Can you work these out from the model? Positions are in its coordinate system, mm. A direction names the side the tool comes from. Coordinates: 2 decimals unless noted, no trailing zeros. Write each loop counter-clockwise with the first axis right and the second up, starting at its lowest first coordinate (ties: lowest second). Pieces come first, ordered by that corner, then holes. Notation, with made-up numbers: (-22.5, 2.5) -> (0.5, 2.5) arc R16 cw to (0.5, 9.5) -> close; hole circle Ø7 at (78, 83.25). An arc over 180 degrees is marked (long way). Answer as CSV lines item,"result". Start each with the question number.
Autodesk Inventor part; units mm, degrees
ref_plane "YZ Plane" through (0, 0, 0) normal (1, 0, 0) x (0, 1, 0)
ref_plane "XZ Plane" through (0, 0, 0) normal (0, 1, 0) x (-1, 0, 0)
ref_plane "XY Plane" through (0, 0, 0) normal (0, 0, 1) x (1, 0, 0)
sketch "Sketch1" plane through (0, 0, 0) normal (0, 1, 0) x (-1, 0, 0)
  circle A0 centre (0, 0) radius 25.4
  dimension "d0" = 50.8
extrude "Extrusion1" add sketch "Sketch1" against normal blind 25.4
fillet "Fillet1" radius 6.35 1 edges at (25.4, -25.4, 0)
hole "Hole1" at (0, -25.4, 0) direction (0, 1, 0) diameter 6.7564 end through all counterbore diameter 11.1252 counterbore depth 6.35
properties part number "foot"
Q1. Which directions (+Z, -Z, +X, -X, +Y, -Y) give clear straight access to the entire face, cutting with the end or side of a thin tool? Please do faces 1 (the face through (-1.671, -22.181, -5.306)), 2 (the face through (-5, 0, 0)).
Q2. If we mould it in two halves opening along X, with no side actions, what happens to faces 3 (the face through (-4, -25.4, 5)), 4 (the face through (5.506, -9.392, -24.796)), 5 (the face through (0, -19.05, -4))? For each: released by +X, released by -X, zero draft, split by the parting line, or undercut.
Q3. I need wall thicknesses on L1, parallel to Z at x = 0, y = -6.75; L2, parallel to Z at x = 2, y = -19.5; L3, parallel to Z at x = 15.5, y = -12.5. Which ranges of each line are inside material? Lowest first, please.
Q4. Imagine slicing it at A-A (z = 0). Write out the boundary of the cut face in (x, y), then the cut area to 3 significant figures.
Q5. Imagine slicing it at C-C (y = -11). Write out the boundary of the cut face in (x, z).
Q6. Imagine slicing it at B-B (x = 0). Write out the boundary of the cut face in (y, z).
Q7. For pin 1 (6 mm diameter, centred on y = -6, z = -13, fed in from -X); pin 2 (1 mm diameter, centred on x = -18.5, z = 16, fed in from +Y); pin 3 (4 mm diameter, centred on x = -14, z = -17.5, fed in from -Y); pin 4 (10 mm diameter, centred on y = -15.5, z = -9, fed in from -X), each with a flat end and sliding along its axis, tell me the tip position at first contact or that it passes through.
Entries:
1,face 1,"-Y"
1,face 2,"+Z, -Z, +X, -X, +Y"
2,face 3,"zero draft"
2,face 4,"split by the parting line"
2,face 5,"undercut"
3,L1,"-25.4 to -3.38, 3.38 to 25.4"
3,L2,"-25.31 to -5.19, 5.19 to 25.31"
3,L3,"-20.12 to 20.12"
4,outline,"(-25.4, -19.05) arc R6.35 ccw to (-19.05, -25.4) -> (-5.56, -25.4) -> (-5.56, -19.05) -> (-3.38, -19.05) -> (-3.38, 0) -> (-25.4, 0) -> close; (3.38, -19.05) -> (5.56, -19.05) -> (5.56, -25.4) -> (19.05, -25.4) arc R6.35 ccw to (25.4, -19.05) -> (25.4, 0) -> (3.38, 0) -> close"
4,area,"1,070 mm2"
5,outline,"circle Ø50.8 at (0, 0); hole circle Ø6.76 at (0, 0)"
6,outline,"(-25.4, -19.05) arc R6.35 ccw to (-19.05, -25.4) -> (0, -25.4) -> (0, -3.38) -> (-19.05, -3.38) -> (-19.05, -5.56) -> (-25.4, -5.56) -> close; (-25.4, 5.56) -> (-19.05, 5.56) -> (-19.05, 3.38) -> (0, 3.38) -> (0, 25.4) -> (-19.05, 25.4) arc R6.35 ccw to (-25.4, 19.05) -> close"
7,pin 1,"x = -23.35"
7,pin 2,"y = 0"
7,pin 3,"y = -25.25"
7,pin 4,"x = -25.08"
